Could you check a few things on this drawing? It's one solid part, dimensions in mm from its lowest x, y, z. A direction names the side the tool comes from. Give positions to 0.01 mm unless a question says otherwise; leave off trailing zeros. Loops run counter-clockwise (first coordinate to the right, second up) from the corner with the lowest first, then second, coordinate; pieces in that order, holes last.
1. Imagine slicing it at C-C (y = 28). List the corners of the cut face in (x, z) for me, plus the area to 3 significant figures.
2. For the marked faces 1 and 2, which set-ups out of +Z, -Z, +X, -X, +Y, -Y let a thin tool reach every point of the face, with its end or its side?
3. Imagine slicing it at A-A (x = 22). List the corners of the cut face in (y, z) for me (1 decimal).
4. Imagine slicing it at D-D (y = 36). List the corners of the cut face in (x, z) for me, plus the area to 3 significant figures.
5. Imagine slicing it at B-B (z = 2.25). List the corners of the cut face in (x, y) for me (1 decimal), plus the area to 3 significant figures.
6. I need wall thicknesses on line 1 along X through (y, z) = (40, 5.45); line 2 along Y through (x, z) = (28.5, 6.25); line 3 along Y through (x, z) = (25.5, 1) (1 decimal). Which ranges of each line are inside material? Lowest first, please.
7. Thinking about a two-plate mould opening in X: for the marked faces 3 and 4, which applies, +X half, -X half, draft (parallel to the pull), parting line (faces both ways), or undercut?
8. For P1, Ø18, axis at x = 25, y = 26.5, coming from the +Z side; P2, Ø3.5, axis at x = 13, z = 11.5, coming from the +Y side; P3, Ø3, axis at x = 14.5, y = 30, coming from the +Z side, each with a flat end and sliding along its axis, tell me the tip position at first contact or that it passes through.
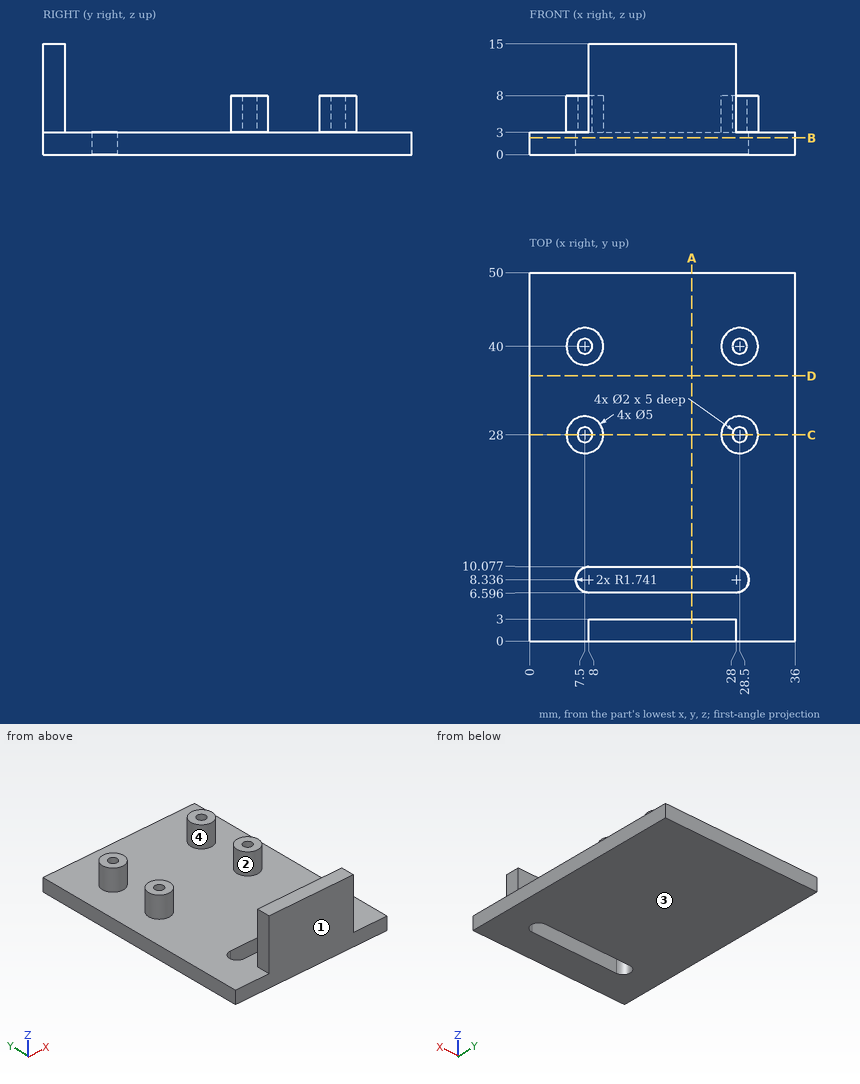
Derived:
1. outline: (0, 0) - (36, 0) - (36, 3) - (31, 3) - (31, 8) - (29.5, 8) - (29.5, 3) - (27.5, 3) - (27.5, 8) - (26, 8) - (26, 3) - (10, 3) - (10, 8) - (8.5, 8) - (8.5, 3) - (6.5, 3) - (6.5, 8) - (5, 8) - (5, 3) - (0, 3) - close
1. area: 138 mm2
2. face 1: +Z, -Z, +X, -X, -Y
2. face 2: +Z
3. outline: (0, 0) - (6.6, 0) - (6.6, 3) - (3, 3) - (3, 15) - (0, 15) - close; (10.1, 0) - (50, 0) - (50, 3) - (10.1, 3) - close
4. outline: (0, 0) - (36, 0) - (36, 3) - (0, 3) - close
4. area: 108 mm2
5. outline: (0, 0) - (36, 0) - (36, 50) - (0, 50) - close; hole (8, 6.6) - (28, 6.6) arc R1.7 ccw to (28, 10.1) - (8, 10.1) arc R1.7 ccw to start
5. area: 1,720 mm2
6. line 1: x = 5 to 6.5, 8.5 to 10, 26 to 27.5, 29.5 to 31
6. line 2: y = 25.5 to 27, 29 to 30.5, 37.5 to 39, 41 to 42.5
6. line 3: y = 0 to 6.6, 10.1 to 50
7. face 3: draft
7. face 4: undercut
8. P1: stops at z = 8
8. P2: stops at y = 3
8. P3: stops at z = 3
